Geometry: see drawing. Coordinates: mm, zero at the bounding-box minimum. A direction names the side the tool comes from. Coordinates: 2 decimals unless noted, no trailing zeros. Loops run counter-clockwise (first coordinate to the right, second up) from the corner with the lowest first, then second, coordinate; pieces in that order, holes last. Notation, with made-up numbers: (19.5, 60) - (46.5, 60) arc R29 cw to (46.5, 82) - close; hole circle Ø3 at (9.25, 56.5). An arc over 180 degrees is marked (long way). Use one line per item in the form item = value.
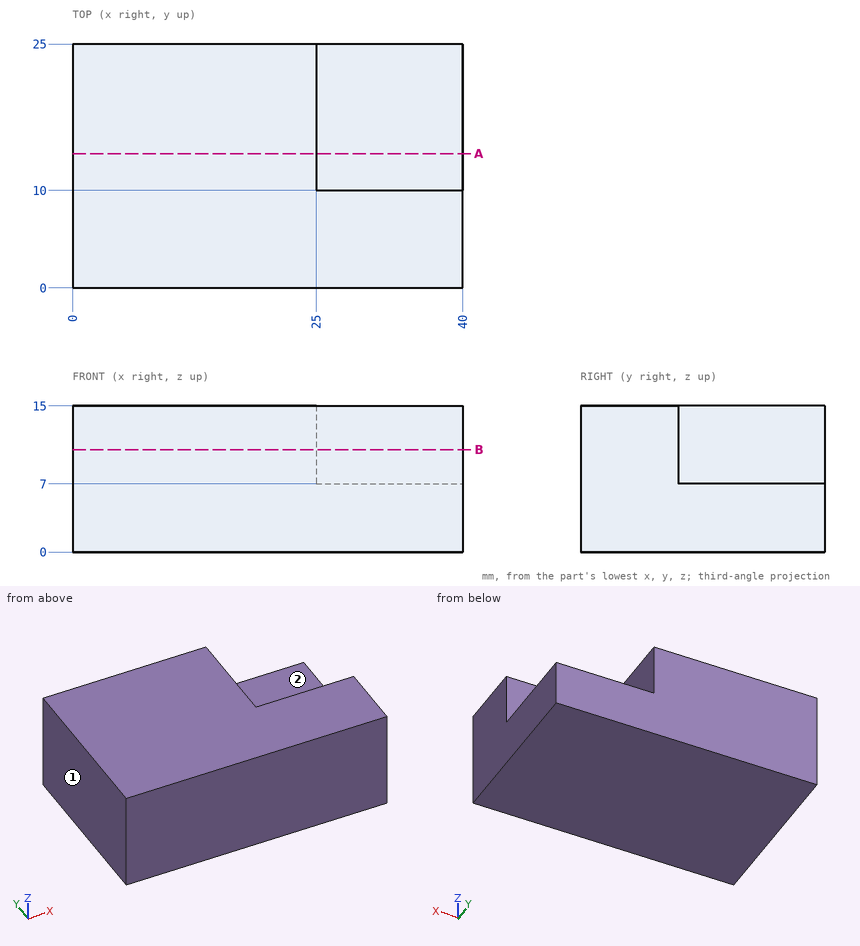
Q1. Set-up query: the marked faces 1 and 2. Return all of +Z, -Z, +X, -X, +Y, -Y with unobstructed straight access to the full face (end or side cutting, diameter ignored); none if empty.
Check values:
face_1 = +Z, -Z, -X, +Y, -Y
face_2 = +Z, +X, +Y
Q2. Ray query, line 1 along Y through (x, z) = (37, 10.5); line 2 along X through (y, z) = (12, 8.5); line 3 along Z through (x, y) = (37, 19.25). Return the intervals inside material, ascending. Write a range as [from, to].
Check values:
line_1 = [0, 10]
line_2 = [0, 25]
line_3 = [0, 7]
Q3. First-contact query: P1, Ø9, axis at x = 35.5, z = 10, coming from the +Y side; P2, Ø6.5, axis at y = 20.5, z = 10.5, coming from the +X side. Flat tips, straight axial feed; report the tip coordinate or a pass-through.
Check values:
P1 = 25
P2 = 25
Q4. Cut plane B-B, the plane z = 10.5. Return loops of the section in (x, y).
Check values:
outline = (0, 0) - (40, 0) - (40, 10) - (25, 10) - (25, 25) - (0, 25) - close
Q5. Cut plane A-A, the plane y = 13.75. Return loops of the section in (x, z).
Check values:
outline = (0, 0) - (40, 0) - (40, 7) - (25, 7) - (25, 15) - (0, 15) - close
